from build123d import *

# Parameters (mm, degrees)
F0_W     = 10
F0_H     = 10
F1_DEPTH = 60
F2_R     = 2.8575
F3_DEPTH = 10.16
F4_R     = 2.8575
F5_DEPTH = 10.16


with BuildPart() as f1:
    # F0 (on Top) → F1 (new body)
    with BuildSketch(Plane.XY):
        Rectangle(F0_W, F0_H)
    extrude(amount=F1_DEPTH)

    # F2 (on Top) → F3 (cut)
    with BuildSketch(Plane.XY):
        Circle(F2_R)
    extrude(amount=F3_DEPTH, mode=Mode.SUBTRACT)

    # F4 (on face) → F5 (cut)
    with BuildSketch(Plane.XY.offset(60)):
        Circle(F4_R)
    extrude(amount=-F5_DEPTH, mode=Mode.SUBTRACT)


solid = f1.part
CAD build for the part. Positions are in the model's coordinates, mm. A direction names the side the tool comes from. Coordinates: 2 decimals unless noted, no trailing zeros. Order: outer loops, then holes, each group sorted by start corner. A loop starts at its lowest first (then second) coordinate and runs counter-clockwise, first axis right, second up. Notation, with made-up numbers: (11.25, 44.5) -> (69.25, 44.5) arc R27 cw to (69.25, 73.5) -> close; hole circle Ø9 at (77.5, 85.5). An arc over 180 degrees is marked (long way). Answer in a Markdown table with one row per item.
1) Band-saw the part on A-A (y = 0). List the corners of the cut face in (x, z).
Check values:
| item | result |
|---|---|
| outline | (-5, 0) -> (-2.86, 0) -> (-2.86, 10.16) -> (2.86, 10.16) -> (2.86, 0) -> (5, 0) -> (5, 60) -> (2.86, 60) -> (2.86, 49.84) -> (-2.86, 49.84) -> (-2.86, 60) -> (-5, 60) -> close |
2) Drill centre lines: line 1 (Y direction, x = 0, z = 55.5); line 2 (Z direction, x = 0.75, y = 0.25); line 3 (Y direction, x = -1, z = 9). Where is each one in solid material? Low to high.
Check values:
| item | result |
|---|---|
| line 1 | -5 to -2.86, 2.86 to 5 |
| line 2 | 10.16 to 49.84 |
| line 3 | -5 to -2.68, 2.68 to 5 |
3) Flat gauge pin, fed straight in: P1, Ø4.5, axis at x = 0, y = 0, coming from the +Z side. Where does the tip first touch, or does it go through?
Check values:
| item | result |
|---|---|
| P1 | z = 49.84 |
4) Band-saw the part on C-C (z = 9.5). List the corners of the cut face in (x, y) (1 decimal), and give its area (3 significant figures).
Check values:
| item | result |
|---|---|
| outline | (-5, -5) -> (5, -5) -> (5, 5) -> (-5, 5) -> close; hole circle Ø5.7 at (0, 0) |
| area | 74.3 mm2 |
5) Which spindle directions (+Z, -Z, +X, -X, +Y, -Y) get a long thin tool onto all of the face, cutting with end or side? Do faces 4 (the face through (2.726, 0.858, 5.009)), 5 (the face through (0, 5, 30)), 6 (the face through (2.726, 0.858, 54.991)). Say none if no direction does.
Check values:
| item | result |
|---|---|
| face 4 | -Z |
| face 5 | +Z, -Z, +X, -X, +Y |
| face 6 | +Z |
6) Mould opens along Y. For faces 1 (the face through (0, 0, 10.16)), 2 (the face through (2.2, 2.3, 60)), 3 (the face through (0, -5, 30)) say: pulls with the +Y half, pulls with the -Y half, needs draft (parallel to the pull), parting line crosses it, or undercut.
Check values:
| item | result |
|---|---|
| face 1 | undercut |
| face 2 | needs draft |
| face 3 | pulls with the -Y half |
